Can you work these out from the model? Positions are in its coordinate system, mm. Face numbers are marked on the shaded views. A direction names the side the tool comes from. Coordinates: 2 decimals unless noted, no trailing zeros. Loops run counter-clockwise (first coordinate to the right, second up) from the corner with the lowest first, then second, coordinate; pieces in that order, holes last. Notation, with made-up numbers: (2, 64.5) - (19, 64.5) arc R19 ccw to (19, 79.5) - close; hole circle Ø2 at (7, 64.5). An arc over 180 degrees is marked (long way). Put each result on its own line as item: value. Start each with the question number.
from build123d import *

# Parameters (mm, degrees)
SKETCH1_W               = 50
SKETCH1_H               = 750
BOSS_EXTRUDE1_DEPTH     = 94
SKETCH2_W               = 70
SKETCH2_H               = 50
BOSS_EXTRUDE2_DEPTH     = 253
SKETCH3_R               = 20
CUT_EXTRUDE1_DEPTH      = 10
CUT_EXTRUDE2_DEPTH      = 537.465549172
CUT_EXTRUDE2_DEPTH_BACK = 537.465549172
SKETCH4_R               = 25


with BuildPart() as part:
    # Sketch1 → Boss-Extrude1 (new body)
    with BuildSketch(Plane(origin=(0, 0, 0), x_dir=(1, 0, 0), z_dir=(0, 1, 0))):
        with Locations((-449.137931034, -133.836206897)):
            Rectangle(SKETCH1_W, SKETCH1_H)
    extrude(amount=BOSS_EXTRUDE1_DEPTH)

    # Sketch2 → Boss-Extrude2 (add)
    with BuildSketch(Plane(origin=(0, 94, 0), x_dir=(1, 0, 0), z_dir=(0, 1, 0))):
        with Locations((-449.137931034, 216.163793103)):
            Rectangle(SKETCH2_W, SKETCH2_H)
        with Locations((-449.137931034, -483.836206897)):
            Rectangle(SKETCH2_W, SKETCH2_H)
    extrude(amount=-BOSS_EXTRUDE2_DEPTH)

    # Sketch3 → Cut-Extrude1 (cut)
    with BuildSketch(Plane.ZY.offset(474.137931034)):
        with Locations((-137.663793103, 47)):
            Circle(SKETCH3_R)
        with Locations((405.336206897, 47)):
            Circle(SKETCH3_R)
    extrude(amount=-CUT_EXTRUDE1_DEPTH, mode=Mode.SUBTRACT)

    # Sketch4 → Cut-Extrude2 (cut, two sides: drawn at the far end of the back side and taken through both)
    with BuildSketch(Plane(origin=(-424.137931034, 0, 0), x_dir=(0, 0, -1), z_dir=(1, 0, 0)).offset(-CUT_EXTRUDE2_DEPTH_BACK)):
        with Locations((-121.436206897, 47)):
            Circle(SKETCH4_R)
    extrude(amount=CUT_EXTRUDE2_DEPTH + CUT_EXTRUDE2_DEPTH_BACK, mode=Mode.SUBTRACT)


solid = part.part
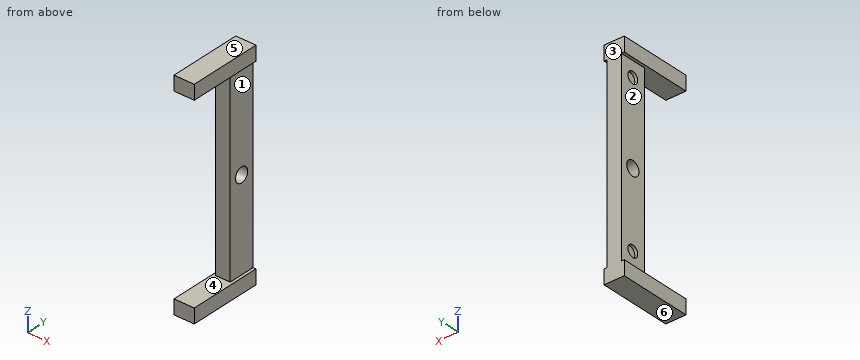
Q1. We'd pull the mould along Z, two halves only. Please class the marked faces 3, 4, 5 and 6: released by +Z, released by -Z, zero draft, split by the parting line, or undercut.
Q2. I want a section at A-A on y = 47. List the corners of the cut face in (x, z) for me, and give its area (3 significant figures).
Q3. I want a section at C-C on y = -51.5. List the corners of the cut face in (x, z) for me, and give its area (3 significant figures).
Q4. I want a section at D-D on z = -140.5. List the corners of the cut face in (x, y) for me.
Q5. I want a section at B-B on x = -433.5. List the corners of the cut face in (y, z) for me.
Q6. On a 3-axis mill with a long thin cutter (end or side, diameter ignored), from which of +Z, -Z, +X, -X, +Y, -Y can I reach the whole of each face in a straight line? I mean the marked faces 1 and 2. Say none if no direction works.
Q7. Will these pins go through, and if not, where does the flat tip stop? pin 1 (15 mm diameter, centred on x = -445, z = 63, fed in from -Y); pin 2 (2 mm diameter, centred on y = 19, z = 151.5, fed in from +X); pin 3 (12 mm diameter, centred on y = 41, z = -143, fed in from -X).
Q8. Please list where these lines run through material, in increasing order: line 1 along Z through (x, y) = (-467, 48.5); line 2 along Z through (x, y) = (-470, -83); line 3 along Y through (x, z) = (-470.5, 405). Write a range as [from, to].
Calculated:
1. face 3: zero draft
1. face 4: undercut
1. face 5: released by +Z
1. face 6: released by -Z
2. outline: (-484.14, -241.16) - (-414.14, -241.16) - (-414.14, -191.16) - (-424.14, -191.16) - (-424.14, 96.44) - (-474.14, 96.44) - (-474.14, -117.66) - (-464.14, -117.66) - (-464.14, -157.66) - (-474.14, -157.66) - (-474.14, -191.16) - (-484.14, -191.16) - close; (-484.14, 458.84) - (-474.14, 458.84) - (-474.14, 425.34) - (-464.14, 425.34) - (-464.14, 385.34) - (-474.14, 385.34) - (-474.14, 146.44) - (-424.14, 146.44) - (-424.14, 458.84) - (-414.14, 458.84) - (-414.14, 508.84) - (-484.14, 508.84) - close
2. area: 36,200 mm2
3. outline: (-484.14, -241.16) - (-414.14, -241.16) - (-414.14, -191.16) - (-484.14, -191.16) - close; (-484.14, 458.84) - (-414.14, 458.84) - (-414.14, 508.84) - (-484.14, 508.84) - close
3. area: 7,000 mm2
4. outline: (-474.14, 0) - (-424.14, 0) - (-424.14, 94) - (-474.14, 94) - (-474.14, 66.8) - (-464.14, 66.8) - (-464.14, 27.2) - (-474.14, 27.2) - close
5. outline: (-159, -241.16) - (94, -241.16) - (94, 508.84) - (-159, 508.84) - (-159, 458.84) - (0, 458.84) - (0, -191.16) - (-159, -191.16) - close; hole circle Ø50 at (47, 121.44)
6. face 1: +X, +Y, -Y
6. face 2: -X, +Y, -Y
7. pin 1: y = 0
7. pin 2: x = -424.14
7. pin 3: x = -464.14
8. line 1: [-241.16, -157.61], [-117.72, 96.48], [146.39, 385.39], [425.28, 508.84]
8. line 2: [-241.16, -191.16], [458.84, 508.84]
8. line 3: [0, 27], [67, 94]
